Source: three-view drawing plus pictorial views. Frame: mm from the lowest corner of the part. A direction names the side the tool comes from. Coordinates: 2 decimals unless noted, no trailing zeros. Order: outer loops, then holes, each group sorted by start corner. A loop starts at its lowest first (then second) coordinate and runs counter-clockwise, first axis right, second up. Notation, with made-up numbers: (11, -18.75) - (31, -18.75) arc R25 cw to (31, 3.25) - close; hole circle Ø10 at (82, 85). An arc over 180 degrees is marked (long way). One line per question, with ' | ' between items.
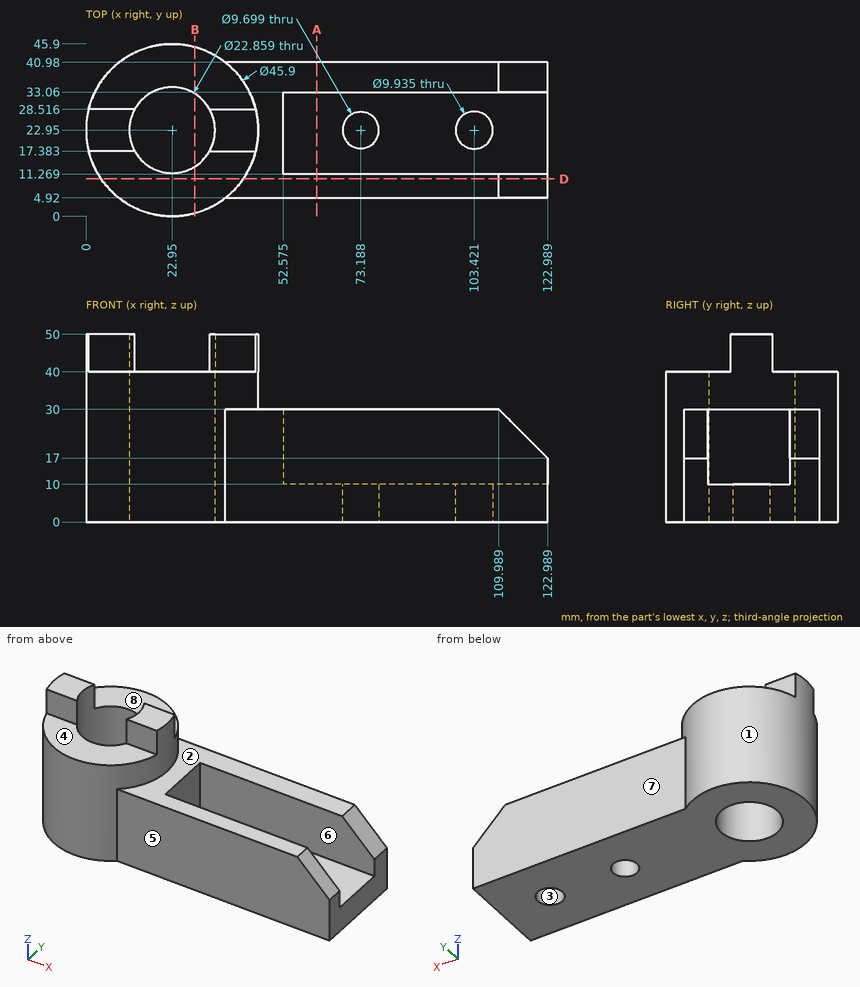
Item 1: Draft query along Y for the marked faces 1, 2 and 3. Return one class per face: released by +Y, released by -Y, zero draft, split by the parting line, or undercut.
Data:
face 1: split by the parting line | face 2: zero draft | face 3: undercut
Item 2: Ray query, line 1 (Y direction, x = 96, z = 29); line 2 (Z direction, x = 107, y = 16); line 3 (X direction, y = 22, z = 23.5) (1 decimal). Return the intervals inside material, ascending.
Data:
line 1: 4.92 to 11.27, 33.06 to 40.98 | line 2: 0 to 10 | line 3: 0 to 11.6, 34.3 to 52.6
Item 3: Contact query for flat-ended pins moving along their axis: P1, Ø15, axis at x = 99, z = 10, coming from the -Y side; P2, Ø5, axis at x = 6, z = 46.5, coming from the +Y side; P3, Ø1, axis at x = 12.5, y = 12.5, coming from the +Z side; P4, Ø13, axis at x = 103.42, y = 22.95, coming from the -Z side. Output: stop coordinate, or through.
Data:
P1: y = 4.92 | P2: y = 28.52 | P3: z = 40 | P4: z = 0
Item 4: Section D-D on y = 10. Return the cut outline in (x, z).
Data:
outline: (4, 0) - (122.99, 0) - (122.99, 17) - (109.99, 30) - (41.9, 30) - (41.9, 40) - (4, 40) - close
Item 5: Section A-A on x = 61.5. Return the cut outline in (y, z), and give its area (3 significant figures).
Data:
outline: (4.92, 0) - (40.98, 0) - (40.98, 30) - (33.06, 30) - (33.06, 10) - (11.27, 10) - (11.27, 30) - (4.92, 30) - close | area: 646 mm^2
Item 6: Access query for the marked faces 4, 5, 6, 7 and 8. Directions: +Z, -Z, +X, -X, +Y, -Y. A direction counts if a zero-diameter tool reaches every point of the face in a straight line with its end or side. Return the directions, or none.
Data:
face 4: +Z, +X, -X, -Y | face 5: +Z, -Z, +X, -Y | face 6: +Z, +X | face 7: +Z, -Z, +X, +Y | face 8: +Z, +X, -X, +Y
Item 7: Section B-B on x = 29. Return the cut outline in (y, z).
Data:
outline: (0.81, 0) - (13.25, 0) - (13.25, 40) - (0.81, 40) - close; (32.65, 0) - (45.09, 0) - (45.09, 40) - (32.65, 40) - close
